The listing builds one solid part. Answer for the finished solid, in the listing's coordinates (mm). Coordinates: 2 decimals unless noted, no trailing zeros. Loops run counter-clockwise (first coordinate to the right, second up) from the corner with the lowest first, then second, coordinate; pieces in that order, holes last. Notation, with made-up numbers: M 64.25,56 L 81.25,56 A11 ccw 81.25,77 Z; hole C 47.25,53 d9. An arc over 180 degrees is marked long. Return JSON: item names as keys, results as strings. Group by question number.
1. The mould has two halves that part along X. Classify faces 1 (the face through (-53.19, -0.96, 4.82)), 2 (the face through (-59.94, 2.64, 4.68)), 3 (the face through (-27, 45, 0)): pulls with the +X half, pulls with the -X half, needs draft (parallel to the pull), parting line crosses it, or undercut.
2. Section A-A (x = 0) is taken. Write down the section's boundary in (y, z), then the cut area to 4 significant figures.
3. Section D-D (x = 27.5) is taken. Write down the section's boundary in (y, z), then the cut area to 3 significant figures.
4. Straight lines are drawn through the part: L1, parallel to Y at x = 0, z = 3.75; L2, parallel to Y at x = 1, z = 8; L3, parallel to Y at x = -27.75, z = 6.25. For each, find the intervals that lie inside material, in ascending order. Write a range as from..to.
5. Section B-B (y = 37) is taken. Write down the section's boundary in (x, z).
6. Section C-C (x = 40) is taken. Write down the section's boundary in (y, z).
7. Given P1, Ø4, axis at x = -43.5, z = 5, coming from the +Y side; P2, Ø4, axis at y = 46, z = 8, coming from the +X side; P3, Ø5, axis at x = -38, z = 3.5, coming from the +Y side; P4, Ø6.5, axis at x = -48.06, y = 27.75, coming from the +Z side, each flat-ended and moving along its own axis, determine where each tip first touches the part or whether it passes through.
```python
from build123d import *

# Parameters (mm, degrees)
ESBO_O1_R                = 60
RESSALTO_EXTRUS_O1_DEPTH = 9.5
ESBO_O2_R                = 51
ESBO_O2_R_2              = 2.5
CORTE_EXTRUS_O1_DEPTH    = 10.5


with BuildPart() as part:
    # Esboço1 → Ressalto-extrusão1 (new body)
    with BuildSketch(Plane.XY):
        Circle(ESBO_O1_R)
    extrude(amount=RESSALTO_EXTRUS_O1_DEPTH)

    # Esboço2 → Corte-extrusão1 (cut, through all)
    with BuildSketch(Plane.XY.offset(9.5)):
        Circle(ESBO_O2_R)
        with Locations((0, 55.5)):
            Circle(ESBO_O2_R_2)
        with Locations((27.75, 48.06440991)):
            Circle(ESBO_O2_R_2)
        with Locations((48.06440991, 27.75)):
            Circle(ESBO_O2_R_2)
        with Locations((55.5, 0)):
            Circle(ESBO_O2_R_2)
        with Locations((48.06440991, -27.75)):
            Circle(ESBO_O2_R_2)
        with Locations((27.75, -48.06440991)):
            Circle(ESBO_O2_R_2)
        with Locations((-27.75, -48.06440991)):
            Circle(ESBO_O2_R_2)
        with Locations((-48.06440991, -27.75)):
            Circle(ESBO_O2_R_2)
        with Locations((-55.5, 0)):
            Circle(ESBO_O2_R_2)
        with Locations((-48.06440991, 27.75)):
            Circle(ESBO_O2_R_2)
        with Locations((-27.75, 48.06440991)):
            Circle(ESBO_O2_R_2)
    extrude(amount=-CORTE_EXTRUS_O1_DEPTH, mode=Mode.SUBTRACT)


solid = part.part
```
Worked out:
{
 "1": {"face 1": "undercut", "face 2": "parting line crosses it", "face 3": "needs draft"},
 "2": {"outline": "M -60,0 L -51,0 L -51,9.5 L -60,9.5 Z; M 51,0 L 53,0 L 53,9.5 L 51,9.5 Z; M 58,0 L 60,0 L 60,9.5 L 58,9.5 Z", "area": "123.5 mm^2"},
 "3": {"outline": "M -53.33,0 L -50.55,0 L -50.55,9.5 L -53.33,9.5 Z; M -45.58,0 L -42.95,0 L -42.95,9.5 L -45.58,9.5 Z; M 42.95,0 L 45.58,0 L 45.58,9.5 L 42.95,9.5 Z; M 50.55,0 L 53.33,0 L 53.33,9.5 L 50.55,9.5 Z", "area": "103 mm^2"},
 "4": {"L1": "-60..-51, 51..53, 58..60", "L2": "-59.99..-50.99, 50.99..53.21, 57.79..59.99", "L3": "-53.2..-50.56, -45.56..-42.79, 42.79..45.56, 50.56..53.2"},
 "5": {"outline": "M -47.23,0 L -35.1,0 L -35.1,9.5 L -47.23,9.5 Z; M 35.1,0 L 47.23,0 L 47.23,9.5 L 35.1,9.5 Z"},
 "6": {"outline": "M -44.72,0 L -31.64,0 L -31.64,9.5 L -44.72,9.5 Z; M 31.64,0 L 44.72,0 L 44.72,9.5 L 31.64,9.5 Z"},
 "7": {"P1": "y = 43.33", "P2": "x = 40.79", "P3": "y = 48.37", "P4": "z = 9.5"}
}
